Autodesk Inventor part; units mm, degrees
ref_plane "YZ Plane" through (0, 0, 0) normal (1, 0, 0) x (0, 1, 0)
ref_plane "XZ Plane" through (0, 0, 0) normal (0, 1, 0) x (-1, 0, 0)
ref_plane "XY Plane" through (0, 0, 0) normal (0, 0, 1) x (1, 0, 0)
sketch "Neo Motor Mount" plane through (0, 0, 0) normal (0, 0, 1) x (1, 0, 0)
  line L0 (-30.6788, 181.9654) -> (-23.3726, 145.6169) construction
  line L1 (-43.3455, 180.5359) -> (-35.6081, 142.0424) construction
  arc A0 (-42.1579, 174.6277) -> (-41.2194, 169.9586) centre (-41.6886, 172.2931) ccw
  line L2 (-35.6081, 142.0424) -> (-32.6003, 127.0788) construction
  line L3 (-23.3726, 145.6169) -> (-20.1494, 129.5815) construction
  arc A1 (-35.0803, 139.4164) -> (-34.1417, 134.7473) centre (-34.611, 137.0818) ccw
  arc A2 (-21.6908, 137.25) -> (-22.6293, 141.9191) centre (-22.16, 139.5845) ccw
  line L4 (-35.0803, 139.4164) -> (-22.6293, 141.9191)
  line L5 (-34.1417, 134.7473) -> (-21.6908, 137.25)
  arc A3 (-77.3692, 167.55) -> (-76.4307, 162.8809) centre (-76.9, 165.2155) ccw
  arc A4 (-63.9797, 165.3836) -> (-64.9183, 170.0527) centre (-64.449, 167.7182) ccw
  arc A5 (-70.2916, 132.3387) -> (-69.3531, 127.6696) centre (-69.8223, 130.0042) ccw
  arc A6 (-56.9021, 130.1723) -> (-57.8406, 134.8414) centre (-57.3714, 132.5069) ccw
  line L6 (-70.2916, 132.3387) -> (-57.8406, 134.8414)
  line L7 (-69.3531, 127.6696) -> (-56.9021, 130.1723)
  line L8 (-77.3692, 167.55) -> (-64.9183, 170.0527)
  line L9 (-76.4307, 162.8809) -> (-63.9797, 165.3836)
  arc A7 (-28.7684, 172.4613) -> (-29.7069, 177.1304) centre (-29.2377, 174.7958) ccw
  line L10 (-42.1579, 174.6277) -> (-29.7069, 177.1304)
  line L11 (-41.2194, 169.9586) -> (-28.7684, 172.4613)
  line L12 (-45.711, 165.6236) -> (-40.743, 140.9077) construction
  line L13 (-58.0667, 162.6468) -> (-53.1939, 138.405) construction
  line L14 (-57.5073, 159.8642) -> (-45.1815, 162.9896)
  line L15 (-53.7533, 141.1877) -> (-41.4275, 144.3131)
  arc A8 (-57.5073, 159.8642) -> (-52.8309, 141.4216) centre (-55.6303, 150.5259) ccw
  arc A9 (-46.2915, 152.4) -> (-46.438, 153.0215) centre (-55.6303, 150.5259) ccw
  arc A10 (-49.53, 157.8411) -> (-51.2107, 158.9635) centre (-55.6303, 150.5259) ccw
  arc A11 (-52.747, 152.4) -> (-52.6427, 151.7743) centre (-43.3045, 153.6514) ccw
  arc A12 (-49.53, 160.8603) -> (-51.2107, 158.9635) centre (-43.3045, 153.6514) ccw
  arc A13 (-41.4275, 144.3131) -> (-46.1039, 162.7557) centre (-43.3045, 153.6514) ccw
  dimension "d55" = 4.7625
  dimension "d57" = 4.7625
  dimension "d58" = 4.7625
  dimension "d61" = 4.7625
  dimension "d62" = 4.7625
  dimension "d63" = 4.7625
  dimension "d64" = 4.7625
  dimension "d65" = 4.7625
  dimension "d67" = 24.7159
sketch "Sketch1" plane through (0, 0, 0) normal (0, 0, 1) x (1, 0, 0)
  line L0 (0, 0) -> (254, 0)
  line L1 (254, 0) -> (254, 355.6)
  line L2 (254, 355.6) -> (0, 355.6)
  line L3 (0, 355.6) -> (-88.9, 355.6)
  line L4 (-88.9, 355.6) -> (-88.9, 203.2)
  line L5 (0, 0) -> (-19.05, 0)
  line L6 (-19.05, 0) -> (-19.05, 76.2)
  line L7 (-19.05, 76.2) -> (-88.9, 76.2)
  line L8 (-88.9, 76.2) -> (-88.9, 203.2)
  circle A0 centre (226.06, 181.61) radius 3.3782
  dimension "d29" = 6.7564
  dimension "d0" = 254
  dimension "d1" = 355.6
  dimension "d17" = 88.9
  dimension "d18" = 69.85
  dimension "d19" = 76.2
  dimension "d21" = 6.7564
  dimension "d24" = 173.99
  dimension "d28" = 314.96
extrude "Extrusion1" add sketch "Sketch1" along normal blind 19.05 contours L5 L6 L7 L8 L4 L3 L2 L1 L0 | A0
sketch "Sketch2" plane through (0, 0, 19.05) normal (0, 0, 1) x (1, 0, 0)
  line L0 (0, 0) -> (254, 0)
  line L1 (254, 0) -> (254, 355.6)
  point P0 (203.2, 203.2)
  dimension "d11" = 203.2
  dimension "d12" = 50.8
hole "Hole1" at (203.2, 203.2, 19.05) direction (0, 0, -1) diameter 28.575 end through all
sketch "Sketch3" plane through (0, 0, 19.05) normal (0, 0, 1) x (1, 0, 0)
  point P0 (0, 0)
sketch "Sketch4" plane through (0, 0, 19.05) normal (0, 0, 1) x (1, 0, 0)
  point P0 (0, 0)
sketch "Sketch5" plane through (0, 0, 0) normal (0, 0, -1) x (-1, 0, 0)
  circle A0 centre (-7.62, 325.12) radius 3.3782
  circle A1 centre (2.54, 133.35) radius 3.3782
  circle A2 centre (-50.8, 40.64) radius 3.3782
  line L0 (-254, 0) -> (-254, 355.6)
  line L1 (-254, 355.6) -> (88.9, 355.6)
  line L2 (88.9, 76.2) -> (19.05, 76.2) construction
  line L3 (19.05, 76.2) -> (19.05, 374.6855) construction
  line L4 (19.05, 76.2) -> (19.05, 0) construction
  line L5 (19.05, 0) -> (-254, 0) construction
  point P0 (0, 0)
  dimension "d29" = 6.7564
  dimension "d30" = 6.7564
  dimension "d31" = 6.7564
  dimension "d32" = 246.38
  dimension "d33" = 256.54
  dimension "d34" = 203.2
  dimension "d35" = 30.48
  dimension "d36" = 222.25
  dimension "d37" = 314.96
  dimension "d40" = 16.51
  dimension "d42" = 26.67
  dimension "d43" = 40.64
  dimension "d44" = 133.35
  dimension "d45" = 325.12
  dimension "d46" = 69.85
extrude "Extrusion2" cut sketch "Sketch5" against normal through all
sketch "Sketch6" plane through (0, 0, 19.05) normal (0, 0, 1) x (1, 0, 0)
  line L0 (-114.6965, 152.4) -> (136.1638, 152.4) construction
  line L1 (-88.9, 355.6) -> (-88.9, 76.2) construction
  line L2 (-88.9, 76.2) -> (-19.05, 76.2) construction
  circle A0 centre (203.2, 203.2) radius 14.2875 construction
  line L3 (-49.53, 152.4) -> (203.2, 203.2) construction
  line L4 (-49.53, 152.4) -> (-245.9533, 112.9179) construction
  line L5 (-49.53, 44.7746) -> (-49.53, 143.2108) construction
  line L6 (-49.53, 146.4424) -> (-49.53, 372.917) construction
  line L7 (-58.0667, 162.6468) -> (-53.1939, 138.405) construction
  line L8 (-45.711, 165.6236) -> (-40.743, 140.9077) construction
  arc A1 (-38.8574, 127.4068) -> (-47.5966, 179.1246) centre (-43.227, 153.2657) ccw
  arc A2 (-60.1251, 177.0076) -> (-51.3859, 125.2897) centre (-55.7555, 151.1486) ccw
  line L9 (-60.1251, 177.0076) -> (-47.5966, 179.1246)
  line L10 (-51.3859, 125.2897) -> (-38.8574, 127.4068)
  point P0 (0, 0)
  point P1 (-57.5073, 159.8642)
  point P2 (-45.1815, 162.9896)
  point P3 (-53.7533, 141.1877)
  point P4 (-41.4275, 144.3131)
  point P5 (-47.5966, 179.1246)
  dimension "d48" = 76.2
  dimension "d83" = 24.7159
extrude "Extrusion4" cut sketch "Sketch6" against normal through all
properties part number "Shaft Mount with NEO mount" material "Wood (Maple)"
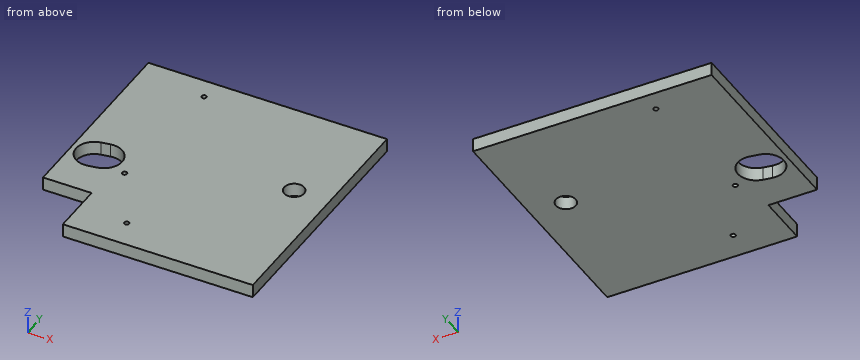
Design review of the part built by this model. Coordinates are the model's own, in mm. Give positions to 0.01 mm unless a question says otherwise; leave off trailing zeros. Order: outer loops, then holes, each group sorted by start corner. A loop starts at its lowest first (then second) coordinate and runs counter-clockwise, first axis right, second up. Notation, with made-up numbers: (78.5, -2) - (133.5, -2) arc R28 cw to (133.5, 28) - close; hole circle Ø9 at (-22.75, 0). An arc over 180 degrees is marked (long way). Use CSV: the item, a comma, the result in double quotes. Start each with the question number.
Q1. Take a section at A-A (x = 203.2). State the section outline as (y, z) points, and give its area (3 significant figures).
Q2. For line 1 (X direction, y = 325.12, z = 10); line 2 (Y direction, x = 203.2, z = 8); line 3 (X direction, y = 133.35, z = 12.5), list the stretches that pass through material, from the lowest coordinate up.
Q3. Take a section at B-B (z = 8.5). Count the separate pieces of the cut face and the enclosed holes in it, and give its area (3 significant figures).
Q4. For P1, Ø10, axis at y = 68, z = 14.5, coming from the -X side; P2, Ø5.5, axis at x = -70, z = 9, coming from the -Y side, all flat-tipped, find the tip position at first contact; note any pin that passes through.
Calculated:
1,outline,"(0, 0) - (188.91, 0) - (188.91, 19.05) - (0, 19.05) - close; (217.49, 0) - (355.6, 0) - (355.6, 19.05) - (217.49, 19.05) - close"
1,area,"6,230 mm²"
2,line 1,"x = -88.9 to 4.24, 11 to 254"
2,line 2,"y = 0 to 188.91, 217.49 to 355.6"
2,line 3,"x = -88.9 to -75.02, -26.16 to -5.92, 0.84 to 254"
3,separate pieces,"1"
3,enclosed holes,"5"
3,area,"113,000 mm²"
4,P1,"stops at x = -19.05"
4,P2,"stops at y = 76.2"
